Verification items for the finished model (mm, model axes). Face numbers are marked on the shaded views. A direction names the side the tool comes from. Give positions to 0.01 mm unless a question says otherwise; leave off trailing zeros. Order: outer loops, then holes, each group sorted by start corner. A loop starts at its lowest first (then second) coordinate and runs counter-clockwise, first axis right, second up. Notation, with made-up numbers: (86.25, 48) -> (133.25, 48) arc R5 ccw to (133.25, 53) -> close; hole circle Ø11 at (-7, 19). An arc over 180 degrees is marked (long way). One line per question, with ' | ' between items. Start each with the question number.
Q1. Section check C-C on x = 18. Record the cut outline in (y, z).
Q2. Material ranges on probe 1 along X at (y, z) = (55.5, 7.5); probe 2 along Z at (x, y) = (-55.5, 28.5); probe 3 along Y at (x, z) = (-29, 34), recorded low to high. Write a range as [from, to].
Q3. Section check A-A on z = 11.5. Record the cut outline in (x, y), plus the area to 3 significant figures.
Q4. Access from +Z, -Z, +X, -X, +Y, -Y to the whole of each face (thin tool, end or side, straight path). Record for the marked faces 1, 2, 3, 4 and 5.
Q5. Section check B-B on y = 34. Record the cut outline in (x, z), plus the area to 3 significant figures.
Q6. Go/stop test with flat-tipped pins: pin 1 (6 mm diameter, centred on x = -32.5, y = -4.5, fed in from +Z); pin 2 (12 mm diameter, centred on x = -24, y = 43, fed in from +Z); pin 3 (8.5 mm diameter, centred on y = -17.5, z = 7, fed in from +X); pin 4 (10 mm diameter, centred on y = 39.5, z = 31, fed in from +X). Record where each tip stops, or that it passes through.
from build123d import *

# Parameters (mm, degrees)
F0_W     = 61.615169
F0_H     = 27.580866
F1_DEPTH = 63.5
F2_DEPTH = 25.4
F4_R     = 6.35


with BuildPart() as f1:
    # F0 (on Front) → F1 (new body, symmetric)
    with BuildSketch(Plane.XZ):
        with Locations((-30.807584, 7.456179)):
            Rectangle(F0_W, F0_H)
    extrude(amount=F1_DEPTH, both=True)

    # F0 (on Front) → F2 (join, symmetric)
    with BuildSketch(Plane.XZ):
        with BuildLine():
            add(Edge.make_bspline(
                [(-61.615169, 21.246612), (-51.106244, 49.939442), (-20.719279, 57.734624), (14.235076, 57.867013)],
                knots=[0, 0, 0, 0, 84.227748, 84.227748, 84.227748, 84.227748], degree=3))
            Line((-61.615169, 21.246612), (0, 21.246612))
            Line((0, 21.246612), (0, 28.003424))
            ThreePointArc((0, 28.003424), (4.263451, 37.58451), (14.235076, 40.831182))
            Line((14.235076, 40.831182), (14.235076, 57.867013))
        make_face()
    extrude(amount=F2_DEPTH, both=True)

    # F0 (on Front) → F3 (revolve)
    with BuildSketch(Plane.XZ):
        Polygon((41.351497, 57.867013), (14.235076, 57.867013), (14.235076, 40.831182), (14.235076, 36.095049), (41.351497, 36.095049), align=None)
    revolve(axis=Axis((14.235076, 0, 46.981031), (0, 0, -1)))

    # F4
    f4_edges = [f1.edges().sort_by_distance(p)[0] for p in [
        (0, -63.5, 7.456179),
        (-61.615169, -63.5, 7.456179),
        (0, 63.5, 7.456179),
        (-61.615169, 63.5, 7.456179),
    ]]
    fillet(f4_edges, radius=F4_R)


solid = f1.part
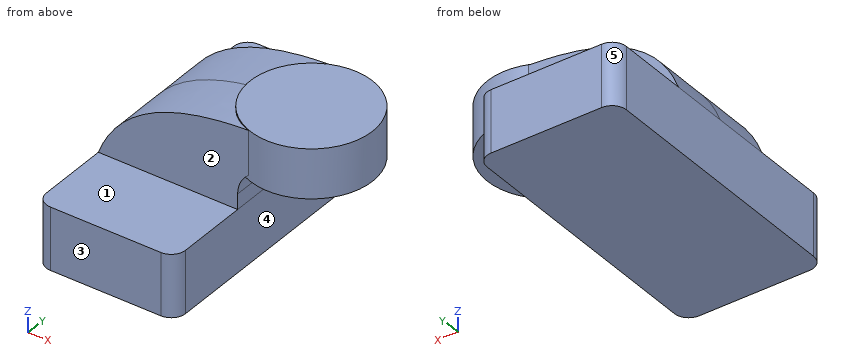
Filled in:
1) outline: (-26.85, 36.1) -> (26.85, 36.1) -> (26.85, 57.87) -> (-26.85, 57.87) -> close
2) probe 1: [-61.62, 0] | probe 2: [-6.33, 21.25] | probe 3: [-25.4, 25.4]
3) outline: (-61.62, -57.15) arc R6.35 ccw to (-55.27, -63.5) -> (-6.35, -63.5) arc R6.35 ccw to (0, -57.15) -> (0, 57.15) arc R6.35 ccw to (-6.35, 63.5) -> (-55.27, 63.5) arc R6.35 ccw to (-61.62, 57.15) -> close | area: 7,790 mm²
4) face 1: +Z, +X, -X, -Y | face 2: +Z, -X, -Y | face 3: +Z, -Z, +X, -X, -Y | face 4: -Z, +X, +Y, -Y | face 5: +Z, -Z, -X, +Y
5) outline: (-61.62, -6.33) -> (0, -6.33) -> (0, 21.25) -> (-61.62, 21.25) -> close | area: 1,700 mm²
6) pin 1: z = 51.57 | pin 2: z = 21.25 | pin 3: x = 0 | pin 4: through
